Verification items for the finished model (mm, model axes). A direction names the side the tool comes from. Give positions to 0.01 mm unless a question says otherwise; leave off trailing zeros. Write each loop counter-clockwise with the first axis right and the second up, starting at its lowest first coordinate (ties: lowest second). Pieces come first, ordered by that corner, then holes. Notation, with made-up numbers: (61, 68.25) -> (98, 68.25) arc R29 ccw to (98, 90.25) -> close; hole circle Ø9 at (70.5, -10.75). An arc over 180 degrees is marked (long way). Answer as CSV lines item,"result".
```python
from build123d import *

# Parameters (mm, degrees)
SKETCH2_R           = 10
BOSS_EXTRUDE1_DEPTH = 0.6
SKETCH3_R           = 7.4
BOSS_EXTRUDE2_DEPTH = 25
SKETCH4_R           = 5
CUT_EXTRUDE1_DEPTH  = 2
SKETCH5_R           = 3
CUT_EXTRUDE2_DEPTH  = 2.5
CUT_EXTRUDE3_DEPTH  = 7


with BuildPart() as part:
    # Sketch2 → Boss-Extrude1 (new body)
    with BuildSketch(Plane.XY):
        Circle(SKETCH2_R)
    extrude(amount=BOSS_EXTRUDE1_DEPTH)

    # Sketch3 → Boss-Extrude2 (add)
    with BuildSketch(Plane(origin=(0, 0, 0), x_dir=(-1, 0, 0), z_dir=(0, 0, -1))):
        Circle(SKETCH3_R)
    extrude(amount=BOSS_EXTRUDE2_DEPTH)

    # Sketch4 → Cut-Extrude1 (cut)
    with BuildSketch(Plane(origin=(0, 0, -25), x_dir=(-1, 0, 0), z_dir=(0, 0, -1))):
        Circle(SKETCH4_R)
    extrude(amount=-CUT_EXTRUDE1_DEPTH, mode=Mode.SUBTRACT)

    # Sketch5 → Cut-Extrude2 (cut)
    with BuildSketch(Plane(origin=(0, 0, -23), x_dir=(-1, 0, 0), z_dir=(0, 0, -1))):
        Circle(SKETCH5_R)
    extrude(amount=-CUT_EXTRUDE2_DEPTH, mode=Mode.SUBTRACT)

    # Sketch6 → Cut-Extrude3 (cut)
    with BuildSketch(Plane(origin=(0, 0, -20.5), x_dir=(-1, 0, 0), z_dir=(0, 0, -1))):
        with BuildLine():
            Line((-2, 2.236067977), (-2, -2.236067977))
            ThreePointArc((-2, -2.236067977), (0, -3), (2, -2.236067977))
            Line((2, -2.236067977), (2, 2.236067977))
            ThreePointArc((2, 2.236067977), (0, 3), (-2, 2.236067977))
        make_face()
    extrude(amount=-CUT_EXTRUDE3_DEPTH, mode=Mode.SUBTRACT)


solid = part.part
```
1) Section check C-C (y = 0). Record the boundary of the cut face in (x, z), and give its area (3 significant figures).
Reported:
outline,"(-10, 0) -> (-7.4, 0) -> (-7.4, -25) -> (-5, -25) -> (-5, -23) -> (-3, -23) -> (-3, -20.5) -> (-2, -20.5) -> (-2, -13.5) -> (2, -13.5) -> (2, -20.5) -> (3, -20.5) -> (3, -23) -> (5, -23) -> (5, -25) -> (7.4, -25) -> (7.4, 0) -> (10, 0) -> (10, 0.6) -> (-10, 0.6) -> close"
area,"319 mm²"
2) Draft check along Y on faces 1 (the flat face through (-5, -2, -25)), 2 (the flat face through (0, 0, -13.5)), 3 (the cylindrical face through (1.604, -7.224, -12.325)). Enter one of: +Y half, -Y half, draft (parallel to the pull), parting line (faces both ways), or undercut.
Reported:
face 1,"draft"
face 2,"undercut"
face 3,"parting line"
3) Scan lines: line 1 along Y through (x, z) = (0, -21.3); line 2 along Z through (x, y) = (2.75, 0.25); line 3 along Z through (x, y) = (2.25, -3.5). Record each from-to range of solid material in increasing order.
Reported:
line 1,"-7.4 to -3, 3 to 7.4"
line 2,"-20.5 to 0.6"
line 3,"-23 to 0.6"
4) Tool access check on faces 4 (the cylindrical face through (-2.17, -9.76, 0.3)), 5 (the flat face through (0.1, -3.3, -23)). Record the directions out of +Z, -Z, +X, -X, +Y, -Y that give a thin tool (end or side, any length) a straight path to the whole face; none if there is none.
Reported:
face 4,"+Z, -Z"
face 5,"-Z"
5) Section check B-B (z = -16.25). Record the boundary of the cut face in (x, y).
Reported:
outline,"circle Ø14.8 at (0, 0); hole (-2, -2.24) arc R3 ccw to (2, -2.24) -> (2, 2.24) arc R3 ccw to (-2, 2.24) -> close"
6) Section check A-A (x = 0). Record the boundary of the cut face in (y, z).
Reported:
outline,"(-10, 0) -> (-7.4, 0) -> (-7.4, -25) -> (-5, -25) -> (-5, -23) -> (-3, -23) -> (-3, -13.5) -> (3, -13.5) -> (3, -23) -> (5, -23) -> (5, -25) -> (7.4, -25) -> (7.4, 0) -> (10, 0) -> (10, 0.6) -> (-10, 0.6) -> close"
7) Section check D-D (z = -7.75). Record the boundary of the cut face in (x, y).
Reported:
outline,"circle Ø14.8 at (0, 0)"
8) Depth check by flat-ended pin: pin 1 (3 mm diameter, centred on x = 0, y = 0, fed in from -Z); pin 2 (10 mm diameter, centred on x = 8, z = -6, fed in from +Y); pin 3 (1.5 mm diameter, centred on x = -0.5, y = -3.5, fed in from -Z). Enter the tip coordinate at first touch or a pass-through.
Reported:
pin 1,"z = -13.5"
pin 2,"y = 6.76"
pin 3,"z = -23"
